Autodesk Inventor part; units mm, degrees
ref_plane "YZ Plane" through (0, 0, 0) normal (1, 0, 0) x (0, 1, 0)
ref_plane "XZ Plane" through (0, 0, 0) normal (0, 1, 0) x (-1, 0, 0)
ref_plane "XY Plane" through (0, 0, 0) normal (0, 0, 1) x (1, 0, 0)
sketch "Sketch2" plane through (0, 0, 0) normal (0, 0, 1) x (1, 0, 0)
  line L0 (22.225, 21.0058) -> (-22.225, 21.0058)
  line L1 (-22.225, 21.0058) -> (-22.225, -21.0058)
  line L2 (-22.225, -21.0058) -> (22.225, -21.0058)
  line L3 (22.225, -21.0058) -> (22.225, 21.0058)
  line L4 (22.225, 21.0058) -> (-22.225, -21.0058) construction
  line L5 (-22.225, 21.0058) -> (22.225, -21.0058) construction
  point P0 (0, 0)
  dimension "d0" = 44.45
  dimension "d1" = 42.0116
extrude "Extrusion1" add sketch "Sketch2" along normal mid plane 3.175
sketch "Sketch3" plane through (0, 0, 1.5875) normal (0, 0, 1) x (1, 0, 0)
  point P0 (0, 0)
  point P1 (0, 0)
hole "Hole1" at (0, 0, 1.5875) direction (0, 0, -1) diameter 28.575 end through all
sketch "Sketch4" plane through (0, 0, 1.5875) normal (0, 0, 1) x (1, 0, 0)
  line L0 (17.9605, -17.9605) -> (-17.9605, 17.9605) construction
  line L1 (-31.115, 0) -> (31.115, 0) construction
  line L2 (0, 29.4081) -> (0, -29.4081) construction
  point P0 (0, 0)
  point P1 (0, 0)
  dimension "d11" = 45
  dimension "d12" = 50.8
hole "Hole2" at (17.9605, -17.9605, 1.5875) at (-17.9605, 17.9605, 1.5875) direction (0, 0, -1) diameter 5.1054 end through all
fillet "Fillet1" radius 3.175 4 edges at (22.225, -21.0058, 0) (-22.225, 21.0058, 0) (22.225, 21.0058, 0) (-22.225, -21.0058, 0)
properties part number "SPACER,NEO550,ARM" material "Nylon 6/6"
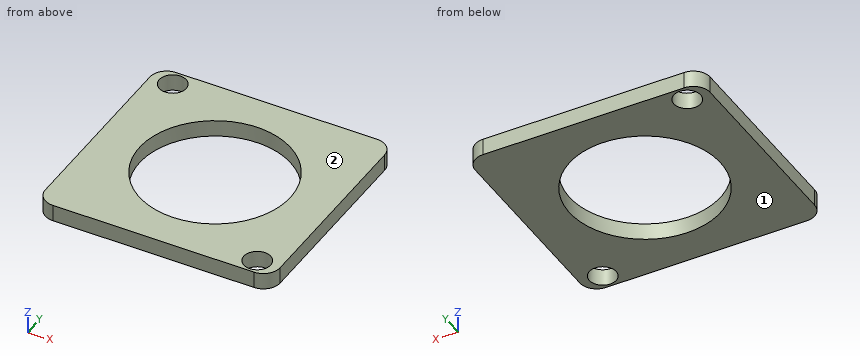
Could you check a few things on this model? Use its own coordinates, in mm. Face numbers are marked on the shaded views. Give positions to 0.01 mm unless a question says otherwise; leave off trailing zeros. Write each loop counter-clockwise with the first axis right and the second up, starting at its lowest first coordinate (ties: lowest second). Pieces come first, ordered by that corner, then holes. Notation, with made-up numbers: (27, 29.25) -> (81, 29.25) arc R20 cw to (81, 58.25) -> close; hole circle Ø2 at (79.25, 61.5). An arc over 180 degrees is marked (long way). Answer as CSV lines item,"result". Start each with the question number.
(1) If we section it at B-B, the plane x = 0: Write out the boundary of the cut face in (y, z), and give its area (3 significant figures).
(2) Please list where these lines run through material, in increasing order: line 1 (Y direction, x = 0, z = 0.35); line 2 (Y direction, x = -10.5, z = -0.35); line 3 (X direction, y = -0.5, z = 0.85) (3 decimals).
(3) If we section it at C-C, the plane z = 1.05: Give the number of separate pieces and of enclosed holes in the cut face, and give its area (3 significant figures).
(4) If we section it at A-A, the plane y = 0: Write out the boundary of the cut face in (x, z) (1 decimal), and give its area (3 significant figures).
(5) If we mould it in two halves opening along Z, with no side actions, what happens to the marked faces 1 and 2? For each: +Z half, -Z half, draft (parallel to the pull), parting line (faces both ways), or undercut.
Answer list:
1,outline,"(-21.01, -1.59) -> (-14.29, -1.59) -> (-14.29, 1.59) -> (-21.01, 1.59) -> close; (14.29, -1.59) -> (21.01, -1.59) -> (21.01, 1.59) -> (14.29, 1.59) -> close"
1,area,"42.7 mm^2"
2,line 1,"-21.01 to -14.29, 14.29 to 21.01"
2,line 2,"-21.01 to -9.69, 9.69 to 21.01"
2,line 3,"-22.225 to -14.279, 14.279 to 22.225"
3,separate pieces,"1"
3,enclosed holes,"3"
3,area,"1,180 mm^2"
4,outline,"(-22.2, -1.6) -> (-14.3, -1.6) -> (-14.3, 1.6) -> (-22.2, 1.6) -> close; (14.3, -1.6) -> (22.2, -1.6) -> (22.2, 1.6) -> (14.3, 1.6) -> close"
4,area,"50.4 mm^2"
5,face 1,"-Z half"
5,face 2,"+Z half"
